from build123d import *

# Parameters (mm, degrees)
CROQUIS3_W              = 51
CROQUIS3_H              = 16
SALIENTE_EXTRUIR1_DEPTH = 8
CORTAR_EXTRUIR4_DEPTH   = 55.046276467
CROQUIS32_R             = 2.5
CORTAR_EXTRUIR6_DEPTH   = 55.046276467


with BuildPart() as part:
    # Croquis3 → Saliente-Extruir1 (new body)
    with BuildSketch(Plane(origin=(0, 0, 0), x_dir=(1, 0, 0), z_dir=(0, 1, 0))):
        with Locations((25.5, 8)):
            Rectangle(CROQUIS3_W, CROQUIS3_H)
    extrude(amount=SALIENTE_EXTRUIR1_DEPTH)

    # Croquis15 → Cortar-Extruir4 (cut, through all)
    with BuildSketch(Plane(origin=(0, 8, 0), x_dir=(1, 0, 0), z_dir=(0, 1, 0))):
        with BuildLine():
            Line((8.5, 11.25), (33, 11.25))
            ThreePointArc((33, 11.25), (36.25, 8), (33, 4.75))
            Line((33, 4.75), (8.5, 4.75))
            ThreePointArc((8.5, 4.75), (5.25, 8), (8.5, 11.25))
        make_face()
    extrude(amount=-CORTAR_EXTRUIR4_DEPTH, mode=Mode.SUBTRACT)

    # Croquis32 → Cortar-Extruir6 (cut, through all)
    with BuildSketch(Plane(origin=(0, 8, 0), x_dir=(1, 0, 0), z_dir=(0, 1, 0))):
        with Locations(Location((44, 8, 0), (0, 0, 270))):
            Circle(CROQUIS32_R)
    extrude(amount=-CORTAR_EXTRUIR6_DEPTH, mode=Mode.SUBTRACT)


solid = part.part
Build history of the part. All positions in model axes, mm. A direction names the side the tool comes from. Give positions to 0.01 mm unless a question says otherwise; leave off trailing zeros. Loops run counter-clockwise (first coordinate to the right, second up) from the corner with the lowest first, then second, coordinate; pieces in that order, holes last. Notation, with made-up numbers: (-21.5, 23.5) -> (-12.5, 23.5) arc R25 ccw to (-12.5, 35.5) -> close; hole circle Ø2 at (51, 78.5). An arc over 180 degrees is marked (long way). Answer in a Markdown table with one row per item.
Item 1: Flat gauge pins, fed straight in: P1, Ø5, axis at x = 32, z = -8.5, coming from the +Y side (3 decimals); P2, Ø6, axis at x = 44, z = -8, coming from the +Y side. Where does each tip first touch, or does it go through?
Findings below:
| item | result |
|---|---|
| P1 | passes through |
| P2 | stops at y = 8 |
Item 2: Probe line 1 along X through (y, z) = (1.5, -8); line 2 along Z through (x, y) = (10, 5.75); line 3 along X through (y, z) = (5.25, -10.25). List the from-to ranges inside material, lowest first. Write a range as [from, to].
Findings below:
| item | result |
|---|---|
| line 1 | x = [0, 5.25], [36.25, 41.5], [46.5, 51] |
| line 2 | z = [-16, -11.25], [-4.75, 0] |
| line 3 | x = [0, 6.15], [35.35, 42.91], [45.09, 51] |
Item 3: Slice it at B-B on z = -8. Write the cut outline in (x, y), plus the area to 3 significant figures.
Findings below:
| item | result |
|---|---|
| outline | (0, 0) -> (5.25, 0) -> (5.25, 8) -> (0, 8) -> close; (36.25, 0) -> (41.5, 0) -> (41.5, 8) -> (36.25, 8) -> close; (46.5, 0) -> (51, 0) -> (51, 8) -> (46.5, 8) -> close |
| area | 120 mm² |
Item 4: Slice it at A-A on x = 26.5. Write the cut outline in (y, z), plus the area to 3 significant figures.
Findings below:
| item | result |
|---|---|
| outline | (0, -16) -> (8, -16) -> (8, -11.25) -> (0, -11.25) -> close; (0, -4.75) -> (8, -4.75) -> (8, 0) -> (0, 0) -> close |
| area | 76.0 mm² |
Item 5: Tool access for faces 4 (the flat face through (0, 4, -8)), 5 (the cylindrical face through (36.25, 4.06, -8.07)): list every direction of +Z, -Z, +X, -X, +Y, -Y with a clear straight run to the whole face (end or side of a thin tool).
Findings below:
| item | result |
|---|---|
| face 4 | +Z, -Z, -X, +Y, -Y |
| face 5 | +Y, -Y |
Item 6: Slice it at C-C on y = 4.5. Write the cut outline in (x, z), plus the area to 3 significant figures.
Findings below:
| item | result |
|---|---|
| outline | (0, -16) -> (51, -16) -> (51, 0) -> (0, 0) -> close; hole (8.5, -11.25) -> (33, -11.25) arc R3.25 ccw to (33, -4.75) -> (8.5, -4.75) arc R3.25 ccw to start; hole circle Ø5 at (44, -8) |
| area | 604 mm² |
Item 7: Slice it at D-D on x = 44. Write the cut outline in (y, z), plus the area to 3 significant figures.
Findings below:
| item | result |
|---|---|
| outline | (0, -16) -> (8, -16) -> (8, -10.5) -> (0, -10.5) -> close; (0, -5.5) -> (8, -5.5) -> (8, 0) -> (0, 0) -> close |
| area | 88.0 mm² |
Item 8: Mould opens along X. For faces 1 (the flat face through (25, 4, 0)), 2 (the flat face through (51, 4, -8)), 3 (the flat face through (21, 4, -4.75)) say: pulls with the +X half, pulls with the -X half, needs draft (parallel to the pull), parting line crosses it, or undercut.
Findings below:
| item | result |
|---|---|
| face 1 | needs draft |
| face 2 | pulls with the +X half |
| face 3 | undercut |
